Could you check a few things on this model? Use its own coordinates, in mm. Face numbers are marked on the shaded views. A direction names the side the tool comes from. Round coordinates to 2 decimals unless told otherwise and drop trailing zeros. Loops run counter-clockwise (first coordinate to the right, second up) from the corner with the lowest first, then second, coordinate; pieces in that order, holes last. Notation, with made-up numbers: M -15,59.5 L 16,59.5 A30 ccw 16,81.5 Z; hole C 26,11.5 d8. An arc over 180 degrees is marked long. Answer in a Markdown table with one row per item.
```python
from build123d import *

# Parameters (mm, degrees)
EXTRUDE_1_DEPTH = 15
SKETCH_3_R      = 1.5
EXTRUDE_2_DEPTH = 30


with BuildPart() as part:
    # 草图2 → 凸台-拉伸1 (new body)
    with BuildSketch(Plane(origin=(0, 0, 0), x_dir=(1, 0, 0), z_dir=(0, 1, 0))):
        with BuildLine():
            Line((-1, 3), (1, 3))
            ThreePointArc((1, 3), (4, 0), (1, -3))
            Line((1, -3), (-1, -3))
            ThreePointArc((-1, -3), (-4, 0), (-1, 3))
        make_face()
    extrude(amount=EXTRUDE_1_DEPTH)

    # 草图3 → 凸台-拉伸2 (add)
    with BuildSketch(Plane(origin=(0, 0, 0), x_dir=(1, 0, 0), z_dir=(0, 1, 0))):
        with Locations(Location((0, 0, 0), (0, 0, 270))):
            Circle(SKETCH_3_R)
    extrude(amount=-EXTRUDE_2_DEPTH)


solid = part.part
```
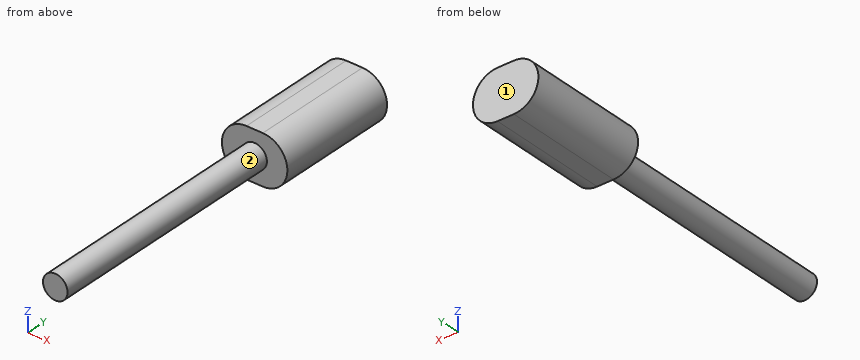
1) I want a section at D-D, the plane x = 3.25. Please give me the cut outline in (y, z).
Computed:
| item | result |
|---|---|
| outline | M 0,-1.98 L 15,-1.98 L 15,1.98 L 0,1.98 Z |
2) I want a section at C-C, the plane y = -15. Please give me the cut outline in (x, z).
Computed:
| item | result |
|---|---|
| outline | C 0,0 d3 |
3) Will these pins go through, and if not, where does the flat tip stop? P1, Ø3, axis at y = -24.5, z = 0, coming from the +X side; P2, Ø1.5, axis at x = 1, y = -19.5, coming from the +Z side; P3, Ø1, axis at x = -2.5, z = 0.5, coming from the -Y side.
Computed:
| item | result |
|---|---|
| P1 | stops at x = 1.5 |
| P2 | stops at z = 1.48 |
| P3 | stops at y = 0 |
4) Which directions (+Z, -Z, +X, -X, +Y, -Y) give clear straight access to the entire face, cutting with the end or side of a thin tool? Please do the marked faces 1 and 2.
Computed:
| item | result |
|---|---|
| face 1 | +Z, -Z, +X, -X, +Y |
| face 2 | -Y |
5) I want a section at A-A, the plane z = 0. Please give me the cut outline in (x, y), plus the area to 3 significant figures.
Computed:
| item | result |
|---|---|
| outline | M -4,0 L -1.5,0 L -1.5,-30 L 1.5,-30 L 1.5,0 L 4,0 L 4,15 L -4,15 Z |
| area | 210 mm² |
6) I want a section at B-B, the plane x = 0. Please give me the cut outline in (y, z), plus the area to 3 significant figures.
Computed:
| item | result |
|---|---|
| outline | M -30,-1.5 L 0,-1.5 L 0,-3 L 15,-3 L 15,3 L 0,3 L 0,1.5 L -30,1.5 Z |
| area | 180 mm² |
7) I need wall thicknesses on line 1 (Y direction, x = 3, z = -1.95); line 2 (X direction, y = 10.5, z = -0.7); line 3 (X direction, y = 5.5, z = 1.7). Which ranges of each line are inside material? Lowest first, please.
Computed:
| item | result |
|---|---|
| line 1 | y = 0 to 15 |
| line 2 | x = -3.92 to 3.92 |
| line 3 | x = -3.47 to 3.47 |
